Part model, mm, in its own coordinate system. Round coordinates to 2 decimals unless told otherwise and drop trailing zeros. Order: outer loops, then holes, each group sorted by start corner. A loop starts at its lowest first (then second) coordinate and runs counter-clockwise, first axis right, second up. Notation, with made-up numbers: (78.25, 82.5) -> (118.25, 82.5) arc R16 ccw to (118.25, 96.5) -> close; hole circle Ø5 at (8.5, -32). An arc over 180 degrees is marked (long way). Use CSV: the item, a comma, the result in double quotes.
```python
from build123d import *

# Parameters (mm, degrees)
RESSALTO_EXTRUS_O1_DEPTH = 3
FILETE1_R                = 6


with BuildPart() as part:
    # Esboço1 → Ressalto-extrusão1 (new body)
    with BuildSketch(Plane.XY):
        with BuildLine():
            Line((306.342806047, -674.493319609), (275.520600999, -674.493319609))
            Line((275.520600999, -674.493319609), (275.520600999, -717.778646353))
            Line((275.520600999, -717.778646353), (233.520600999, -717.778646353))
            ThreePointArc((233.520600999, -717.778646353), (192.534924195, -734.755469548), (175.558100999, -775.741146353))
            Line((175.558100999, -775.741146353), (175.558100999, -817.741146353))
            Line((175.558100999, -817.741146353), (133.558100999, -817.741146353))
            Line((133.558100999, -817.741146353), (133.558100999, -607.741146353))
            Line((133.558100999, -607.741146353), (-270.272488906, -607.741146353))
            Line((-270.272488906, -607.741146353), (-270.272488906, -817.741146353))
            Line((-270.272488906, -817.741146353), (-312.272488906, -817.741146353))
            Line((-312.272488906, -817.741146353), (-312.272488906, -775.741146353))
            ThreePointArc((-312.272488906, -775.741146353), (-329.249312101, -734.755469548), (-370.234988906, -717.778646353))
            Line((-370.234988906, -717.778646353), (-412.234988906, -717.778646353))
            Line((-412.234988906, -717.778646353), (-412.234988906, -674.493319609))
            Line((-412.234988906, -674.493319609), (-443.057193953, -674.493319609))
            Line((-443.057193953, -674.493319609), (-443.057193953, -271.188973097))
            Line((-443.057193953, -271.188973097), (-412.234988906, -271.188973097))
            Line((-412.234988906, -271.188973097), (-412.234988906, -227.903646353))
            Line((-412.234988906, -227.903646353), (-370.234988906, -227.903646353))
            ThreePointArc((-370.234988906, -227.903646353), (-329.249312101, -210.926823158), (-312.272488906, -169.941146353))
            Line((-312.272488906, -169.941146353), (-312.272488906, -127.941146353))
            Line((-312.272488906, -127.941146353), (-270.272488906, -127.941146353))
            Line((-270.272488906, -127.941146353), (-269.391871615, -127.941146353))
            Line((-269.391871615, -127.941146353), (-269.391871615, -97.941146353))
            Line((-269.391871615, -97.941146353), (132.677483708, -97.941146353))
            Line((132.677483708, -97.941146353), (132.677483708, -127.941146353))
            Line((132.677483708, -127.941146353), (133.558100999, -127.941146353))
            Line((133.558100999, -127.941146353), (175.558100999, -127.941146353))
            Line((175.558100999, -127.941146353), (175.558100999, -169.941146353))
            ThreePointArc((175.558100999, -169.941146353), (192.534924195, -210.926823158), (233.520600999, -227.903646353))
            Line((233.520600999, -227.903646353), (275.520600999, -227.903646353))
            Line((275.520600999, -227.903646353), (275.520600999, -271.188973097))
            Line((275.520600999, -271.188973097), (306.342806047, -271.188973097))
            Line((306.342806047, -271.188973097), (306.342806047, -674.493319609))
        make_face()
    extrude(amount=RESSALTO_EXTRUS_O1_DEPTH)

    # Filete1
    filete1_edges = [part.edges().sort_by_distance(p)[0] for p in [
        (306.342806047, -674.493319609, 1.5),
        (275.520600999, -674.493319609, 1.5),
        (275.520600999, -717.778646353, 1.5),
        (175.558100999, -817.741146353, 1.5),
        (133.558100999, -817.741146353, 1.5),
        (133.558100999, -607.741146353, 1.5),
        (-270.272488906, -607.741146353, 1.5),
        (-270.272488906, -817.741146353, 1.5),
        (-312.272488906, -817.741146353, 1.5),
        (-412.234988906, -717.778646353, 1.5),
        (-412.234988906, -674.493319609, 1.5),
        (-443.057193953, -674.493319609, 1.5),
        (-443.057193953, -271.188973097, 1.5),
        (-412.234988906, -271.188973097, 1.5),
        (-412.234988906, -227.903646353, 1.5),
        (-312.272488906, -127.941146353, 1.5),
        (-269.391871615, -127.941146353, 1.5),
        (-269.391871615, -97.941146353, 1.5),
        (132.677483708, -97.941146353, 1.5),
        (175.558100999, -127.941146353, 1.5),
        (275.520600999, -227.903646353, 1.5),
        (275.520600999, -271.188973097, 1.5),
        (306.342806047, -271.188973097, 1.5),
    ]]
    fillet(filete1_edges, radius=FILETE1_R)


solid = part.part
```
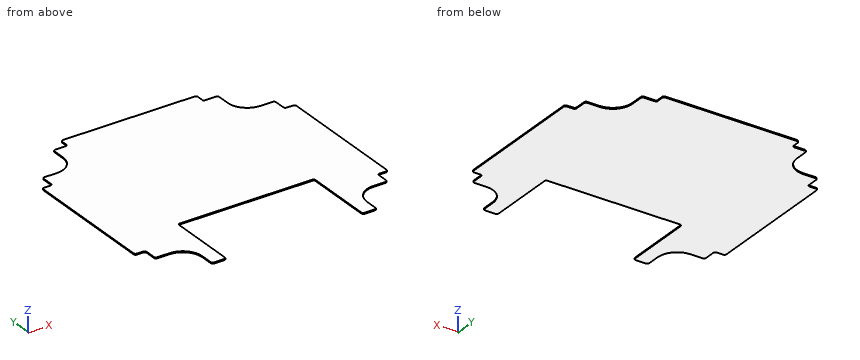
(1) Drop flat-ended pins along their axis: P1, Ø0.9, axis at y = -787.5, z = 1.5, coming from the -X side; P2, Ø1.5, axis at x = 288, z = 1.5, coming from the +Y side; P3, Ø1.5, axis at y = -702.5, z = 1, coming from the +X side. Give the stop position or say it passes through.
Reply:
P1,"x = -312.27"
P2,"y = -271.19"
P3,"x = 275.52"
(2) Cut at B-B, the plane y = -157. Give the cut face in (x, z), then the cut area to 3 significant figures.
Reply:
outline,"(-312.27, 0) -> (175.56, 0) -> (175.56, 3) -> (-312.27, 3) -> close"
area,"1,460 mm2"
(3) Probe probe 1 along Y at (x, z) = (-243, 2.1); probe 2 along Y at (x, z) = (-379, 0.45); probe 3 along X at (y, z) = (-166, 0.15). List the from-to ranges inside material, lowest first. Write a range as [from, to].
Reply:
probe 1,"[-607.74, -97.94]"
probe 2,"[-717.78, -227.9]"
probe 3,"[-312.27, 175.56]"
(4) Cut at A-A, the plane x = -122. Give the cut face in (y, z).
Reply:
outline,"(-607.74, 0) -> (-97.94, 0) -> (-97.94, 3) -> (-607.74, 3) -> close"
